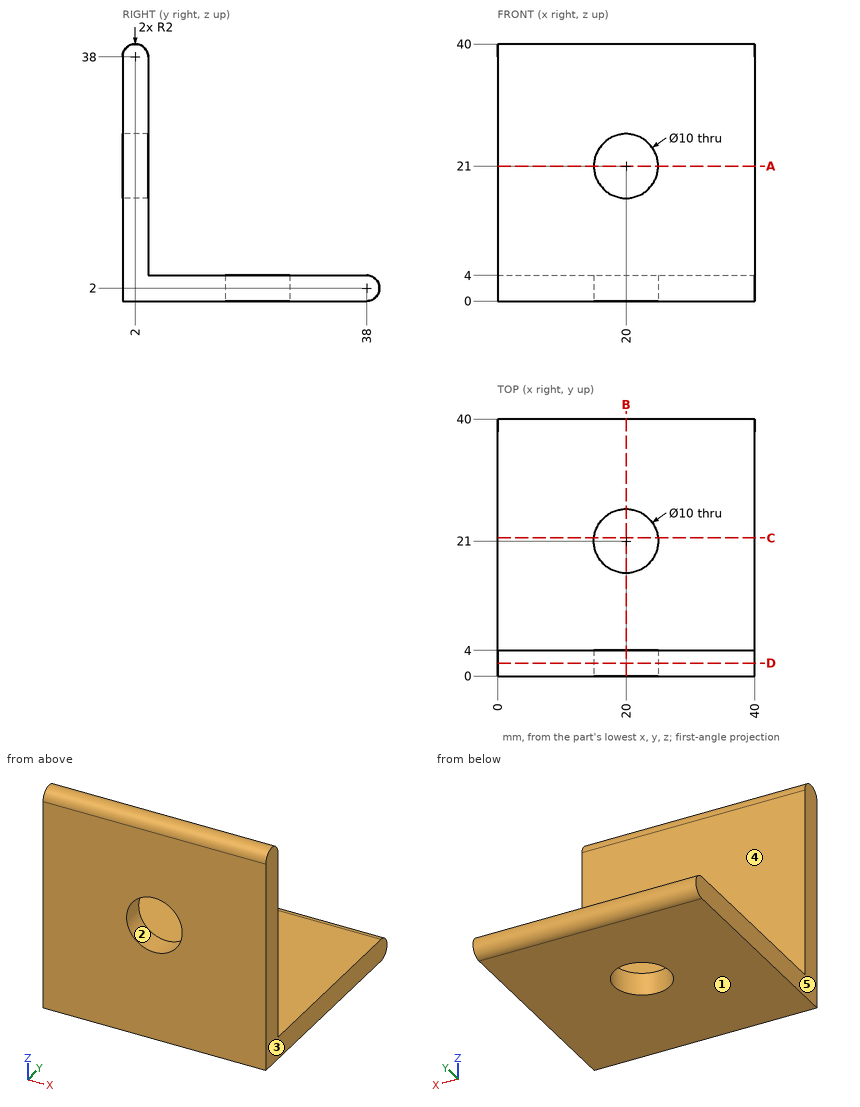
Verification items for this drawing (mm, ordinates from the low corner). A direction names the side the tool comes from. Give positions to 0.01 mm unless a question says otherwise; leave off trailing zeros. Loops run counter-clockwise (first coordinate to the right, second up) from the corner with the lowest first, then second, coordinate; pieces in that order, holes last. Notation, with made-up numbers: M 68,30 L 99,30 A27 cw 99,66 Z; hole C 29,77 d9. An arc over 180 degrees is marked long. Return JSON: item names as keys, results as strings. Group by question number.
1. Cross-section at D-D on y = 2. Record the boundary of the cut face in (x, z).
2. Cross-section at B-B on x = 20. Record the boundary of the cut face in (y, z), plus the area to 3 significant figures.
3. Cross-section at C-C on y = 21.5. Record the boundary of the cut face in (x, z), plus the area to 3 significant figures.
4. Tool access check on the marked faces 4 and 5. Record the directions out of +Z, -Z, +X, -X, +Y, -Y that give a thin tool (end or side, any length) a straight path to the whole face; none if there is none.
5. Cross-section at A-A on z = 21. Record the boundary of the cut face in (x, y).
6. Thickness scan on L1, parallel to Z at x = 20, y = 2; L2, parallel to X at y = 2, z = 21; L3, parallel to Y at x = 38, z = 36. Record the ranges inside material, lowest first.
7. Go/stop test with flat-tipped pins: pin 1 (6 mm diameter, centred on x = 28.5, z = 26.5, fed in from +Y); pin 2 (12 mm diameter, centred on x = 13, y = 12.5, fed in from +Z). Record where each tip stops, or that it passes through.
8. Mould release check, pull along Z, two halves, no side actions. Record for the marked faces 1, 2 and 3: released by +Z, released by -Z, zero draft, split by the parting line, or undercut.
Return value:
{
 "1": {"outline": "M 0,0 L 40,0 L 40,40 L 0,40 Z; hole C 20,21 d10"},
 "2": {"outline": "M 0,0 L 16,0 L 16,4 L 4,4 L 4,16 L 0,16 Z; M 0,26 L 4,26 L 4,38 A2 ccw 0,38 Z; M 26,0 L 38,0 A2 ccw 38,4 L 26,4 Z", "area": "221 mm^2"},
 "3": {"outline": "M 0,0 L 15.03,0 L 15.03,4 L 0,4 Z; M 24.97,0 L 40,0 L 40,4 L 24.97,4 Z", "area": "120 mm^2"},
 "4": {"face 4": "+Z, +X, -X, +Y", "face 5": "+Z, -Z, -X, +Y, -Y"},
 "5": {"outline": "M 0,0 L 15,0 L 15,4 L 0,4 Z; M 25,0 L 40,0 L 40,4 L 25,4 Z"},
 "6": {"L1": "0 to 16, 26 to 40", "L2": "0 to 15, 25 to 40", "L3": "0 to 4"},
 "7": {"pin 1": "y = 4", "pin 2": "z = 4"},
 "8": {"face 1": "released by -Z", "face 2": "undercut", "face 3": "zero draft"}
}
